Source: CAD feature listing. Evaluate the final solid. Frame: model axes, mm. A direction names the side the tool comes from. Round coordinates to 2 decimals unless told otherwise and drop trailing zeros. Loops run counter-clockwise (first coordinate to the right, second up) from the corner with the lowest first, then second, coordinate; pieces in that order, holes last.
(1) Section B-B, the plane z = 0. Return the cut outline in (x, y), plus the area to 3 significant figures.
(2) Material intervals for probe 1 along X at (y, z) = (5.75, 0); probe 2 along X at (y, z) = (5, 2); probe 3 along Z at (x, y) = (-56.5, 3.25), sorted ascending.
(3) Set-up query: faces 4 (the flat face through (-52, 0, -2)), 5 (the cylindrical face through (15.77, 6.218, 50.076)). Return all of +Z, -Z, +X, -X, +Y, -Y with unobstructed straight access to the full face (end or side cutting, diameter ignored); none if empty.
(4) Mould query, pull axis Z, two halves, no side actions, for faces 1 (the flat face through (-112.776, 4, 2)), 2 (the flat face through (-46.4, 4.775, -11.9)), 3 (the flat face through (-2, 4, 112.776)). Classes: pulls with the +Z half, pulls with the -Z half, needs draft (parallel to the pull), parting line crosses it, or undercut.
(5) Section C-C, the plane y = 6.25. Return the cut outline in (x, z).
(6) Section A-A, the plane x = 0. Return the cut outline in (y, z), plus the area to 3 significant figures.
```python
from build123d import *

# Parameters (mm, degrees)
SKETCH1_W           = 225.552
SKETCH1_H           = 225.552
SKETCH1_R           = 52.5
SKETCH1_R_2         = 60
SKETCH1_R_3         = 47.7502
SKETCH1_R_4         = 40
BOSS_EXTRUDE1_DEPTH = 7.62
CUT_EXTRUDE1_START  = 7.62
SKETCH1_4_R         = 52.5
SKETCH1_4_R_2       = 47.7502
CUT_EXTRUDE1_DEPTH  = 2.8448
CIRPATTERN1_COUNT   = 16


with BuildPart() as part:
    # Sketch1 → Boss-Extrude1 (new body)
    with BuildSketch(Plane(origin=(0, 0, 0), x_dir=(1, 0, 0), z_dir=(0, 1, 0))):
        Rectangle(SKETCH1_W, SKETCH1_H)
        Circle(SKETCH1_R, mode=Mode.SUBTRACT)
        Circle(SKETCH1_R_2)
        Circle(SKETCH1_R, mode=Mode.SUBTRACT)
        Circle(SKETCH1_R)
        Circle(SKETCH1_R_3, mode=Mode.SUBTRACT)
        Circle(SKETCH1_R_3)
        with Locations(Location((0, 0, 0), (0, 0, 90))):
            Circle(SKETCH1_R_4, mode=Mode.SUBTRACT)
    extrude(amount=BOSS_EXTRUDE1_DEPTH)

    # Sketch1_4 → Cut-Extrude1 (cut)
    with BuildSketch(Plane(origin=(0, 0, 0), x_dir=(1, 0, 0), z_dir=(0, 1, 0)).offset(CUT_EXTRUDE1_START)):
        with Locations(Location((0, 0, 0), (0, 0, 270))):
            Circle(SKETCH1_4_R)
        with Locations(Location((0, 0, 0), (0, 0, 270))):
            Circle(SKETCH1_4_R_2, mode=Mode.SUBTRACT)
    extrude(amount=-CUT_EXTRUDE1_DEPTH, mode=Mode.SUBTRACT)

    # Sketch4 → M5x0.8 Tapped Hole2 (revolve, cut)
    with BuildSketch(Plane(origin=(55.432771951, 7.62, -22.961005942), x_dir=(0, 0, 1), z_dir=(1, 0, 0))):
        Polygon((0, 0), (0, 13.6618073), (2.1, 12.4), (2.1, 0), align=None)
    m5x0_8_tapped_hole2 = revolve(axis=Axis((55.432771951, 13.97, -22.961005942), (0, -1, 0)), mode=Mode.SUBTRACT)

    # CirPattern1: M5x0.8 Tapped Hole2 ×16 about axis, 12 skipped
    cirpattern1_axis = Axis((0, 7.62, 0), (0, 1, 0))
    add([m5x0_8_tapped_hole2.rotate(cirpattern1_axis, i * 360 / CIRPATTERN1_COUNT) for i in range(1, CIRPATTERN1_COUNT) if i not in (1, 2, 3, 4, 5, 7, 9, 10, 11, 12, 13, 15)], mode=Mode.SUBTRACT)


solid = part.part
```
Output values:
1. outline: (-112.78, 0) - (-40, 0) - (-40, 7.62) - (-47.75, 7.62) - (-47.75, 4.78) - (-52.5, 4.78) - (-52.5, 7.62) - (-112.78, 7.62) - close; (40, 0) - (112.78, 0) - (112.78, 7.62) - (52.5, 7.62) - (52.5, 4.78) - (47.75, 4.78) - (47.75, 7.62) - (40, 7.62) - close
1. area: 1,080 mm2
2. probe 1: x = -112.78 to -52.5, -47.75 to -40, 40 to 47.75, 52.5 to 112.78
2. probe 2: x = -112.78 to -52.46, -47.71 to -39.95, 39.95 to 47.71, 52.46 to 112.78
2. probe 3: z = -112.78 to -24.77, -21.15 to 21.15, 24.77 to 112.78
3. face 4: +Z, -Z, +X, -X, -Y
3. face 5: +Y
4. face 1: needs draft
4. face 2: undercut
4. face 3: pulls with the +Z half
5. outline: (-112.78, -112.78) - (112.78, -112.78) - (112.78, 112.78) - (-112.78, 112.78) - close; circle Ø95.5 at (0, 0); hole circle Ø4.2 at (-55.43, -22.96); hole circle Ø4.2 at (-55.43, 22.96); hole circle Ø105 at (0, 0); hole circle Ø80 at (0, 0); hole circle Ø4.2 at (55.43, -22.96); hole circle Ø4.2 at (55.43, 22.96)
6. outline: (0, -112.78) - (7.62, -112.78) - (7.62, -52.5) - (4.78, -52.5) - (4.78, -47.75) - (7.62, -47.75) - (7.62, -40) - (0, -40) - close; (0, 40) - (7.62, 40) - (7.62, 47.75) - (4.78, 47.75) - (4.78, 52.5) - (7.62, 52.5) - (7.62, 112.78) - (0, 112.78) - close
6. area: 1,080 mm2
